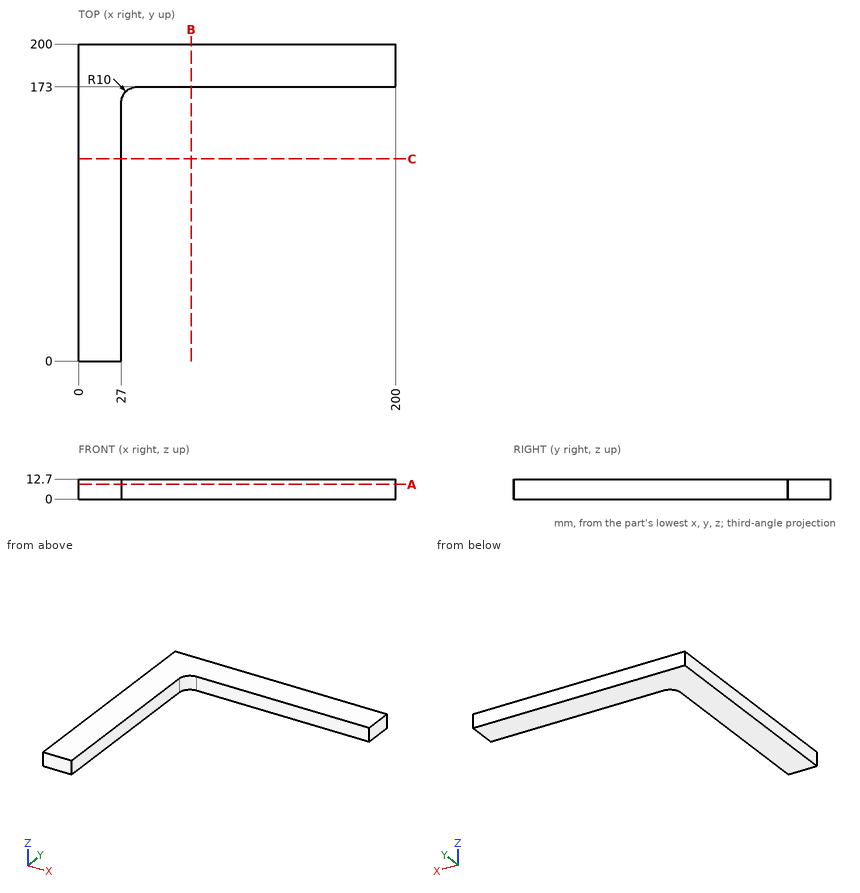
Geometry: see drawing. Coordinates: mm, zero at the bounding-box minimum. Coordinates: 2 decimals unless noted, no trailing zeros. Order: outer loops, then holes, each group sorted by start corner. A loop starts at its lowest first (then second) coordinate and runs counter-clockwise, first axis right, second up. Notation, with made-up numbers: M 44.25,14.5 L 59.25,14.5 A20 ccw 59.25,23.5 Z; hole C -35.5,51 d4. An arc over 180 degrees is marked long. Write each question's results on one line, items separated by ' | '. Start each with the question number.
1) Section query A-A (z = 9.25). Return the cut outline in (x, y), plus the area to 3 significant figures.
2) Contact query for a flat-ended pin moving along its axis: pin 1 Ø4 at (y, z) = (107, 8) entering from +X. Output: stop coordinate, or through.
3) Section query B-B (x = 71). Return the cut outline in (y, z).
4) Line query: line 1 (X direction, y = 109, z = 5.25); line 2 (Y direction, x = 103, z = 7.75); line 3 (X direction, y = 167, z = 3.75). Output: solid intervals per line, ascending. Write a range as from..to.
5) Section query C-C (y = 127.5). Return the cut outline in (x, z), plus the area to 3 significant figures.
Answers:
1) outline: M 0,0 L 27,0 L 27,163 A10 cw 37,173 L 200,173 L 200,200 L 0,200 Z | area: 10,100 mm^2
2) pin 1: stops at x = 27
3) outline: M 173,0 L 200,0 L 200,12.7 L 173,12.7 Z
4) line 1: x = 0..27 | line 2: y = 173..200 | line 3: x = 0..27.83
5) outline: M 0,0 L 27,0 L 27,12.7 L 0,12.7 Z | area: 343 mm^2
